Design review of the part built by this model. Coordinates are the model's own, in mm. A direction names the side the tool comes from. Give positions to 0.01 mm unless a question says otherwise; leave off trailing zeros. Loops run counter-clockwise (first coordinate to the right, second up) from the corner with the lowest first, then second, coordinate; pieces in that order, holes last. Notation, with made-up numbers: M -17.75,87.25 L 36.25,87.25 A9 cw 36.25,99.25 Z; hole C 79,-28 d2. An arc over 180 degrees is marked long. Use CSV: the item, a comma, the result in double quotes.
from build123d import *

# Parameters (mm, degrees)
SKETCH1_W               = 117
SKETCH1_H               = 72
BOSS_EXTRUDE1_DEPTH     = 2.5
SKETCH2_W               = 117
SKETCH2_H               = 72
SKETCH2_W_2             = 110.5
SKETCH2_H_2             = 67
BOSS_EXTRUDE2_DEPTH     = 60
SKETCH3_R               = 1.25
BOSS_EXTRUDE3_DEPTH     = 36
CUT_EXTRUDE1_DEPTH      = 94.884237229
CUT_EXTRUDE1_DEPTH_BACK = 94.884237229
SKETCH4_W               = 15
SKETCH4_H               = 4


with BuildPart() as part:
    # Sketch1 → Boss-Extrude1 (new body)
    with BuildSketch(Plane(origin=(0, 0, 0), x_dir=(1, 0, 0), z_dir=(0, 1, 0))):
        Rectangle(SKETCH1_W, SKETCH1_H)
    extrude(amount=-BOSS_EXTRUDE1_DEPTH)

    # Sketch2 → Boss-Extrude2 (add)
    with BuildSketch(Plane(origin=(0, 0, 0), x_dir=(1, 0, 0), z_dir=(0, 1, 0))):
        Rectangle(SKETCH2_W, SKETCH2_H)
        with Locations((0.75, 0)):
            Rectangle(SKETCH2_W_2, SKETCH2_H_2, mode=Mode.SUBTRACT)
    extrude(amount=BOSS_EXTRUDE2_DEPTH)

    # Sketch3 → Boss-Extrude3 (add, symmetric)
    with BuildSketch(Plane.XY):
        with BuildLine():
            Line((-58.5, 62), (-58.5, 60))
            Line((-58.5, 60), (-54.5, 60))
            Line((-54.5, 60), (-54.5, 62))
            ThreePointArc((-54.5, 62), (-56.5, 64), (-58.5, 62))
        make_face()
        with Locations((-56.5, 62)):
            Circle(SKETCH3_R, mode=Mode.SUBTRACT)
    extrude(amount=BOSS_EXTRUDE3_DEPTH, both=True)

    # Sketch4 → Cut-Extrude1 (cut, two sides: drawn at the far end of the back side and taken through both)
    with BuildSketch(Plane(origin=(0, 0, 0), x_dir=(0, 0, -1), z_dir=(1, 0, 0)).offset(-CUT_EXTRUDE1_DEPTH_BACK)):
        with Locations((-14.5, 62)):
            Rectangle(SKETCH4_W, SKETCH4_H)
        with Locations((14.5, 62)):
            Rectangle(SKETCH4_W, SKETCH4_H)
    extrude(amount=CUT_EXTRUDE1_DEPTH + CUT_EXTRUDE1_DEPTH_BACK, mode=Mode.SUBTRACT)


solid = part.part
(1) Clearance check with flat-ended pins moving along their axes: P1, Ø1.2, axis at x = -56.5, y = 62.5, coming from the +Z side; P2, Ø21.5, axis at x = -2.5, z = 16, coming from the +Y side; P3, Ø1.2, axis at x = -57, z = 18, coming from the +Y side. State where each tip first meets the part, or that it passes through.
A:
P1,"through"
P2,"y = 0"
P3,"y = 60"
(2) We need section C-C on z = -2. State the section outline as (x, y) points, then the cut area to 3 significant figures.
A:
outline,"M -58.5,-2.5 L 58.5,-2.5 L 58.5,60 L 56,60 L 56,0 L -54.5,0 L -54.5,62 A2 ccw -58.5,62 Z; hole C -56.5,62 d2.5"
area,"692 mm²"
(3) We need section A-A on x = -56.5. State the section outline as (y, z) points, then the cut area to 3 significant figures.
A:
outline,"M -2.5,-36 L 60.75,-36 L 60.75,-22 L 60,-22 L 60,-7 L 60.75,-7 L 60.75,7 L 60,7 L 60,22 L 60.75,22 L 60.75,36 L -2.5,36 Z; M 63.25,-36 L 64,-36 L 64,-22 L 63.25,-22 Z; M 63.25,-7 L 64,-7 L 64,7 L 63.25,7 Z; M 63.25,22 L 64,22 L 64,36 L 63.25,36 Z"
area,"4,560 mm²"
(4) We need section D-D on z = 11. State the section outline as (x, y) points, then the cut area to 4 significant figures.
A:
outline,"M -58.5,-2.5 L 58.5,-2.5 L 58.5,60 L 56,60 L 56,0 L -54.5,0 L -54.5,60 L -58.5,60 Z"
area,"682.5 mm²"
(5) We need section B-B on y = 44.5. State the section outline as (x, z) points.
A:
outline,"M -58.5,-36 L 58.5,-36 L 58.5,36 L -58.5,36 Z; hole M -54.5,-33.5 L 56,-33.5 L 56,33.5 L -54.5,33.5 Z"
(6) Wall thickness on line 1 along X through (y, z) = (6.5, -11.5); line 2 along Z through (x, y) = (49, 49.5); line 3 along X through (y, z) = (62, 29): over which ranges is each line inside the solid? List them lowest first. Write a range as [from, to].
A:
line 1,"[-58.5, -54.5], [56, 58.5]"
line 2,"[-36, -33.5], [33.5, 36]"
line 3,"[-58.5, -57.75], [-55.25, -54.5]"
(7) The part is to be moulded in two halves that separate along Y. For faces 6 (the flat face through (-1, 31, 36)), 7 (the flat face through (-1, -2.5, -1)), 8 (the cylindrical face through (-55.828, 63.054, 28.902)), say which applies: released by +Y, released by -Y, zero draft, split by the parting line, or undercut.
A:
face 6,"zero draft"
face 7,"released by -Y"
face 8,"undercut"
(8) Machinability: for faces 1 (the flat face through (0, 30, -33.5)), 2 (the flat face through (18, 60, 34)), 3 (the cylindrical face through (-55.828, 63.054, -29.098)), 4 (the flat face through (-56.1, 60.6, 22)), 5 (the cylindrical face through (-56.5, 64, -28.9)), which of the approach directions +Z, -Z, +X, -X, +Y, -Y give a long, thin tool a straight path to every point of the face, cutting with its end or side? Answer none if there is none.
A:
face 1,"+Y"
face 2,"+Z, -Z, +X, +Y"
face 3,"+Z, -Z"
face 4,"+X, -X, +Y"
face 5,"+Z, -Z, +Y"
